Build history of the part. All positions in model axes, mm. A direction names the side the tool comes from. Give positions to 0.01 mm unless a question says otherwise; leave off trailing zeros. Order: outer loops, then holes, each group sorted by start corner. A loop starts at its lowest first (then second) coordinate and runs counter-clockwise, first axis right, second up. Notation, with made-up numbers: (8, -32.75) - (29, -32.75) arc R25 cw to (29, -12.75) - close; hole circle Ø8 at (26.25, -19.5). An arc over 180 degrees is marked (long way). Use a Markdown table: item, result. Add a question column.
(1) Which spindle directions (+Z, -Z, +X, -X, +Y, -Y) get a long thin tool onto all of the face, cutting with end or side? Do faces 1 (the face through (160.03, 157.88, 5.44)), 2 (the face through (80, 167.4, 0.8)), 3 (the face through (48, 155, 9.5)). Say none if no direction does.
(2) Slice it at C-C (y = 196). Write the cut outline in (x, z).
(3) Slice it at A-A (y = 177). Write the cut outline in (x, z), then the cut area to 3 significant figures.
(4) Slice it at D-D (z = 3.5). Write the cut outline in (x, y), then the cut area to 3 significant figures.
(5) Wall check: line 1 (X direction, y = 212, z = 1); line 2 (Y direction, x = 121.5, z = 1); line 3 (Z direction, x = 124, y = 230.5). Give the ranges that are in metal, low to high.
(6) Slice it at B-B (x = 96). Write the cut outline in (y, z), then the cut area to 3 significant figures.
(7) Flat gauge pin, fed straight in: pin 1 (0.7 mm diameter, centred on x = 47.5, y = 156, fed in from +Z). Where does the tip first touch, or does it go through?
(8) Mould opens along X. For faces 4 (the face through (117, 197, 0)), 5 (the face through (150.12, 237.45, 0.76)) say: +X half, -X half, draft (parallel to the pull), parting line (faces both ways), or undercut.
from build123d import *

# Parameters (mm, degrees)
SKETCH1_W           = 140
SKETCH1_H           = 93.753760253
BOSS_EXTRUDE1_DEPTH = 1.5
SKETCH2_R           = 1.6
CUT_EXTRUDE1_DEPTH  = 1.5
SKETCH3_R           = 2.737611944
SKETCH3_R_2         = 1.237611944
BOSS_EXTRUDE2_DEPTH = 8
SKETCH4_R           = 1.3
SKETCH4_R_2         = 1.35
SKETCH4_R_3         = 1.5875
CUT_EXTRUDE2_DEPTH  = 8
CUT_EXTRUDE3_DEPTH  = 10


with BuildPart() as part:
    # Sketch1 → Boss-Extrude1 (new body)
    with BuildSketch(Plane.XY):
        with Locations((102, 196.095777869)):
            Rectangle(SKETCH1_W, SKETCH1_H)
    extrude(amount=BOSS_EXTRUDE1_DEPTH)

    # Sketch2 → Cut-Extrude1 (cut)
    with BuildSketch(Plane.XY.offset(1.5)):
        with Locations((47.04400772, 240.027868216)):
            Circle(SKETCH2_R)
        with Locations((162.04400772, 240.027868216)):
            Circle(SKETCH2_R)
    extrude(amount=-CUT_EXTRUDE1_DEPTH, mode=Mode.SUBTRACT)

    # Sketch3 → Boss-Extrude2 (add)
    # profile 1 of 2: a face of its own
    with BuildSketch(Plane.XY.offset(1.5)):
        with Locations((47.04400772, 156.027868216)):
            Circle(SKETCH3_R)
        with Locations((47.04400772, 156.027868216)):
            Circle(SKETCH3_R_2, mode=Mode.SUBTRACT)
    # profile 2 of 2: a face of its own
    with BuildSketch(Plane.XY.offset(1.5)):
        with Locations((162.04400772, 156.027868216)):
            Circle(SKETCH3_R)
        with Locations((162.04400772, 156.027868216)):
            Circle(SKETCH3_R_2, mode=Mode.SUBTRACT)
    extrude(amount=BOSS_EXTRUDE2_DEPTH)

    # Sketch4 → Cut-Extrude2 (cut)
    with BuildSketch(Plane(origin=(0, 0, 0), x_dir=(-1, 0, 0), z_dir=(0, 0, -1))):
        with Locations((-120.431826709, 209.617216317)):
            Circle(SKETCH4_R)
        with Locations((-62.434035172, 209.111077258)):
            Circle(SKETCH4_R_2)
        with Locations((-62.861635411, 160.112943028)):
            Circle(SKETCH4_R_2)
        with Locations((-120.859426949, 160.619082087)):
            Circle(SKETCH4_R_2)
        with Locations((-131.613133958, 181.551872542)):
            Circle(SKETCH4_R_3)
        with Locations((-136.693133958, 233.621872542)):
            Circle(SKETCH4_R_3)
        with Locations((-164.633133958, 233.621872542)):
            Circle(SKETCH4_R_3)
    extrude(amount=-CUT_EXTRUDE2_DEPTH, mode=Mode.SUBTRACT)

    # Sketch5 → Cut-Extrude3 (cut)
    with BuildSketch(Plane.XY.offset(1.5)):
        with BuildLine():
            Line((87.370025241, 227.627019548), (87.370025241, 174.953532483))
            ThreePointArc((87.370025241, 174.953532483), (79.813693114, 167.397200355), (72.257360986, 174.953532483))
            Line((72.257360986, 174.953532483), (72.257360986, 227.627019548))
            ThreePointArc((72.257360986, 227.627019548), (79.813693114, 235.183351676), (87.370025241, 227.627019548))
        make_face()
        with BuildLine():
            Line((107.076686064, 226.935622361), (107.076686064, 174.953532483))
            ThreePointArc((107.076686064, 174.953532483), (99.520353936, 167.397200355), (91.964021808, 174.953532483))
            Line((91.964021808, 174.953532483), (91.964021808, 226.935622361))
            ThreePointArc((91.964021808, 226.935622361), (99.520353936, 234.491954489), (107.076686064, 226.935622361))
        make_face()
        with BuildLine():
            Line((142.731512272, 205.818600592), (142.731512272, 229.897268949))
            ThreePointArc((142.731512272, 229.897268949), (150.2878444, 237.453601077), (157.844176528, 229.897268949))
            Line((157.844176528, 229.897268949), (157.844176528, 205.818600592))
            ThreePointArc((157.844176528, 205.818600592), (150.2878444, 198.262268464), (142.731512272, 205.818600592))
        make_face()
        with BuildLine():
            Line((157.844176528, 183.436532175), (157.844176528, 171.821347981))
            ThreePointArc((157.844176528, 171.821347981), (150.2878444, 164.265015853), (142.731512272, 171.821347981))
            Line((142.731512272, 171.821347981), (142.731512272, 183.436532175))
            ThreePointArc((142.731512272, 183.436532175), (150.2878444, 190.992864302), (157.844176528, 183.436532175))
        make_face()
        with BuildLine():
            Line((55.134626412, 225.825721278), (55.134626412, 173.152234213))
            ThreePointArc((55.134626412, 173.152234213), (47.578294284, 165.595902085), (40.021962156, 173.152234213))
            Line((40.021962156, 173.152234213), (40.021962156, 225.825721278))
            ThreePointArc((40.021962156, 225.825721278), (47.578294284, 233.382053406), (55.134626412, 225.825721278))
        make_face()
    extrude(amount=-CUT_EXTRUDE3_DEPTH, mode=Mode.SUBTRACT)


solid = part.part
Solution:
| question | item | result |
|---|---|---|
| 1 | face 1 | +Z |
| 1 | face 2 | +Z, -Z |
| 1 | face 3 | +Z, +X, -X, +Y, -Y |
| 2 | outline | (32, 0) - (40.02, 0) - (40.02, 1.5) - (32, 1.5) - close; (55.13, 0) - (72.26, 0) - (72.26, 1.5) - (55.13, 1.5) - close; (87.37, 0) - (91.96, 0) - (91.96, 1.5) - (87.37, 1.5) - close; (107.08, 0) - (172, 0) - (172, 1.5) - (107.08, 1.5) - close |
| 3 | outline | (32, 0) - (40.02, 0) - (40.02, 1.5) - (32, 1.5) - close; (55.13, 0) - (72.26, 0) - (72.26, 1.5) - (55.13, 1.5) - close; (87.37, 0) - (91.96, 0) - (91.96, 1.5) - (87.37, 1.5) - close; (107.08, 0) - (142.73, 0) - (142.73, 1.5) - (107.08, 1.5) - close; (157.84, 0) - (172, 0) - (172, 1.5) - (157.84, 1.5) - close |
| 3 | area | 119 mm2 |
| 4 | outline | circle Ø5.48 at (47.04, 156.03); circle Ø5.48 at (162.04, 156.03); hole circle Ø2.48 at (47.04, 156.03); hole circle Ø2.48 at (162.04, 156.03) |
| 4 | area | 37.5 mm2 |
| 5 | line 1 | 32 to 40.02, 55.13 to 72.26, 87.37 to 91.96, 107.08 to 142.73, 157.84 to 172 |
| 5 | line 2 | 149.22 to 159.43, 161.81 to 208.88, 210.36 to 242.97 |
| 5 | line 3 | 0 to 1.5 |
| 6 | outline | (149.22, 0) - (168.27, 0) - (168.27, 1.5) - (149.22, 1.5) - close; (233.62, 0) - (242.97, 0) - (242.97, 1.5) - (233.62, 1.5) - close |
| 6 | area | 42.6 mm2 |
| 7 | pin 1 | z = 1.5 |
| 8 | face 4 | draft |
| 8 | face 5 | undercut |
